```python
from build123d import *

# Parameters (mm, degrees)
SKETCH2_W           = 10
SKETCH2_H           = 3.175
BOSS_EXTRUDE1_DEPTH = 3.175


with BuildPart() as part:
    # Sketch2 → Boss-Extrude1 (new body)
    with BuildSketch(Plane(origin=(0, 0, 0), x_dir=(1, 0, 0), z_dir=(0, 1, 0))):
        Polygon((11.456556246, -72.927322323), (111.456556246, -72.927322323), (111.456556246, -62.927322323), (114.631556246, -62.927322323), (114.631556246, -52.927322323), (111.456556246, -52.927322323), (111.456556246, 7.072677677), (114.631556246, 7.072677677), (114.631556246, 17.072677677), (111.456556246, 17.072677677), (111.456556246, 27.072677677), (11.456556246, 27.072677677), (11.456556246, 17.072677677), (8.281556246, 17.072677677), (8.281556246, 7.072677677), (11.456556246, 7.072677677), (11.456556246, -52.927322323), (8.281556246, -52.927322323), (8.281556246, -62.927322323), (11.456556246, -62.927322323), align=None)
        with Locations((26.456556246, 22.310177677)):
            Rectangle(SKETCH2_W, SKETCH2_H, mode=Mode.SUBTRACT)
        with Locations((96.456556246, 22.310177677)):
            Rectangle(SKETCH2_W, SKETCH2_H, mode=Mode.SUBTRACT)
        with Locations((96.456556246, -68.164822323)):
            Rectangle(SKETCH2_W, SKETCH2_H, mode=Mode.SUBTRACT)
        with Locations((26.456556246, -68.164822323)):
            Rectangle(SKETCH2_W, SKETCH2_H, mode=Mode.SUBTRACT)
    extrude(amount=BOSS_EXTRUDE1_DEPTH)


solid = part.part
```
Geometry check sheet. Reference: the model listing, model coordinates, mm. A direction names the side the tool comes from. Give positions to 0.01 mm unless a question says otherwise; leave off trailing zeros. Loops run counter-clockwise (first coordinate to the right, second up) from the corner with the lowest first, then second, coordinate; pieces in that order, holes last. Notation, with made-up numbers: (-11, 54) - (27, 54) arc R18 cw to (27, 76) - close; hole circle Ø4 at (25, -11). An arc over 180 degrees is marked (long way). Use CSV: the item, a comma, the result in double quotes. Start each with the question number.
Q1. Section check B-B, the plane z = 27. Record the cut outline in (x, y) (3 decimals), and give its area (4 significant figures).
Q2. Access from +Z, -Z, +X, -X, +Y, -Y to the whole of each face (thin tool, end or side, straight path). Record for faces 1 (the face through (11.457, 2, -22)), 2 (the face through (21.457, 2, -22)), 3 (the face through (113, 2, -17.073)).
Q3. Go/stop test with flat-tipped pins: pin 1 Ø1 at (y, z) = (1.5, -21.5) entering from +X; pin 2 Ø1.6 at (x, y) = (10.5, 2) entering from +Z. Record where each tip stops, or that it passes through.
Q4. Section check A-A, the plane y = 2.55. Count the separate pieces of the cut face and the enclosed holes in it, and give its area (3 significant figures).
Q5. Release check for a two-part mould opening along X. For faces 4 (the face through (111.457, 2, 68)), 5 (the face through (91.457, 2, -22)), 6 (the face through (11.457, 2, 23)), 7 (the face through (61, 0, 22)) record: +X half, -X half, draft (parallel to the pull), parting line (faces both ways), or undercut.
Q6. Scan lines: probe 1 along Z at (x, y) = (92.5, 0.4); probe 2 along X at (y, z) = (0.7, 31.5). Record each from-to range of solid material in increasing order. Write a range as from..to.
Findings below:
1,outline,"(11.457, 0) - (111.457, 0) - (111.457, 3.175) - (11.457, 3.175) - close"
1,area,"317.5 mm^2"
2,face 1,"-Z, -X, +Y, -Y"
2,face 2,"+Y, -Y"
2,face 3,"-Z, +X, +Y, -Y"
3,pin 1,"stops at x = 111.46"
3,pin 2,"stops at z = 62.93"
4,separate pieces,"1"
4,enclosed holes,"4"
4,area,"10,000 mm^2"
5,face 4,"+X half"
5,face 5,"undercut"
5,face 6,"-X half"
5,face 7,"draft"
6,probe 1,"z = -27.07..-23.9, -20.72..66.58, 69.75..72.93"
6,probe 2,"x = 11.46..111.46"
